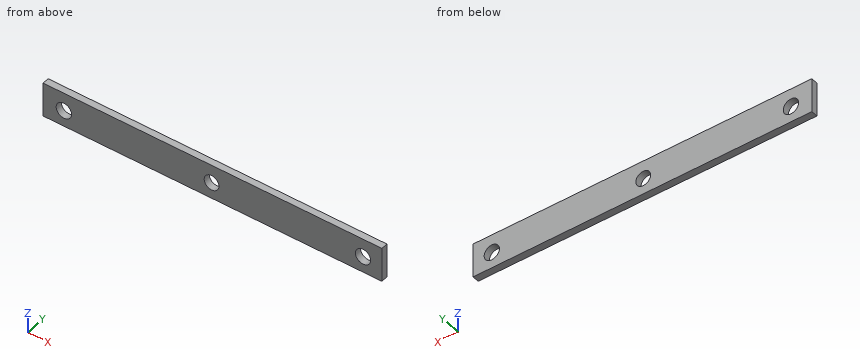
from build123d import *

# Parameters (mm, degrees)
F0_W     = 254
F0_H     = 25.4
F1_DEPTH = 2.54
F2_R     = 5.765709
F2_R_2   = 5.719151
F3_DEPTH = 38.1
F4_R     = 5.551244
F5_DEPTH = 25.4


with BuildPart() as f1:
    # F0 (on Front) → F1 (new body, symmetric)
    with BuildSketch(Plane.XZ):
        with Locations((0.620032, 0.783191)):
            Rectangle(F0_W, F0_H)
    extrude(amount=F1_DEPTH, both=True)

    # F2 (on face) → F3 (cut)
    with BuildSketch(Plane.XZ.offset(2.54)):
        with Locations((-110.739939, 0)):
            Circle(F2_R)
        with Locations((113.527127, 0)):
            Circle(F2_R_2)
    extrude(amount=-F3_DEPTH, mode=Mode.SUBTRACT)

    # F4 (on face) → F5 (cut)
    with BuildSketch(Plane.XZ.offset(2.54)):
        Circle(F4_R)
    extrude(amount=-F5_DEPTH, mode=Mode.SUBTRACT)


solid = f1.part
Verification items for the finished model (mm, model axes). Coordinates: 2 decimals unless noted, no trailing zeros. Loops run counter-clockwise (first coordinate to the right, second up) from the corner with the lowest first, then second, coordinate; pieces in that order, holes last. Notation, with made-up numbers: (66, 34.25) -> (73, 34.25) arc R27 ccw to (73, 73.25) -> close; hole circle Ø11 at (67, 50.25). An arc over 180 degrees is marked (long way). Write each question's results on one line, items separated by ' | '.
Item 1: Section check B-B, the plane z = 0. Enter the section's corners in (x, y).
Found:
outline: (-126.38, -2.54) -> (-116.51, -2.54) -> (-116.51, 2.54) -> (-126.38, 2.54) -> close; (-104.97, -2.54) -> (-5.55, -2.54) -> (-5.55, 2.54) -> (-104.97, 2.54) -> close; (5.55, -2.54) -> (107.81, -2.54) -> (107.81, 2.54) -> (5.55, 2.54) -> close; (119.25, -2.54) -> (127.62, -2.54) -> (127.62, 2.54) -> (119.25, 2.54) -> close
Item 2: Section check A-A, the plane y = 0.4. Enter the section's corners in (x, z).
Found:
outline: (-126.38, -11.92) -> (127.62, -11.92) -> (127.62, 13.48) -> (-126.38, 13.48) -> close; hole circle Ø11.53 at (-110.74, 0); hole circle Ø11.1 at (0, 0); hole circle Ø11.44 at (113.53, 0)
Item 3: Gauge pin test, flat end, axial feed: pin 1 (13.5 mm diameter, centred on x = -110.74, z = 0, fed in from +Y). Record the tip position at first contact, or that the pin passes through.
Found:
pin 1: stops at y = 2.54
Item 4: Section check C-C, the plane x = 0. Enter the section's corners in (y, z), plus the area to 3 significant figures.
Found:
outline: (-2.54, -11.92) -> (2.54, -11.92) -> (2.54, -5.55) -> (-2.54, -5.55) -> close; (-2.54, 5.55) -> (2.54, 5.55) -> (2.54, 13.48) -> (-2.54, 13.48) -> close | area: 72.6 mm2
Item 5: Section check D-D, the plane x = 110.5. Enter the section's corners in (y, z).
Found:
outline: (-2.54, -11.92) -> (2.54, -11.92) -> (2.54, -4.85) -> (-2.54, -4.85) -> close; (-2.54, 4.85) -> (2.54, 4.85) -> (2.54, 13.48) -> (-2.54, 13.48) -> close
Item 6: Material ranges on L1, parallel to X at y = 0.5, z = 0.25; L2, parallel to Z at x = 0, y = -0.4; L3, parallel to X at y = 1, z = 3.5, recorded low to high.
Found:
L1: x = -126.38 to -116.5, -104.98 to -5.55, 5.55 to 107.81, 119.24 to 127.62 | L2: z = -11.92 to -5.55, 5.55 to 13.48 | L3: x = -126.38 to -115.32, -106.16 to -4.31, 4.31 to 109, 118.05 to 127.62
